```python
from build123d import *

# Parameters (mm, degrees)
ESQUISSE1_W                    = 60
ESQUISSE1_H                    = 35
MAIN_DEPTH                     = 3
ESQUISSE2_W                    = 60
ESQUISSE2_H                    = 2.9
HORIZONTALMAKERBEAMRAIL1_DEPTH = 1
ESQUISSE3_R                    = 1.5
VERTICALFIXHOLE_DEPTH          = 5
ESQUISSE4_W                    = 25
ESQUISSE4_H                    = 25
ESQUISSE4_W_2                  = 18
ESQUISSE4_H_2                  = 18
URGENCYBUTTON_DEPTH            = 20
ESQUISSE5_W                    = 18
ESQUISSE5_H                    = 18
URGENCYBUTTONHOLE_DEPTH        = 1
URGENCYBUTTONHOLE_DEPTH_BACK   = 24
BOSS_EXTRU_4_DEPTH             = 5
ESQUISSE7_W                    = 6
ESQUISSE7_H                    = 25
BOSS_EXTRU_5_DEPTH             = 5
ESQUISSE8_W                    = 29.5
ESQUISSE8_H                    = 10.5
SWITCHHOLE_DEPTH               = 29
ESQUISSE10_W                   = 35
ESQUISSE10_H                   = 16.5
ESQUISSE10_W_2                 = 29.5
ESQUISSE10_H_2                 = 10.5
BOSS_EXTRU_6_DEPTH             = 18
ESQUISSE11_W                   = 35
ESQUISSE11_H                   = 8.5
ENL_V_MAT_EXTRU_4_DEPTH        = 4
ESQUISSE12_W                   = 60
ESQUISSE12_H                   = 2.8
BOSS_EXTRU_7_DEPTH             = 1
BOSS_EXTRU_8_DEPTH             = 60
BOSS_EXTRU_9_DEPTH             = 60


with BuildPart() as part:
    # Esquisse1 → Main (new body)
    with BuildSketch(Plane.XY):
        Rectangle(ESQUISSE1_W, ESQUISSE1_H)
    extrude(amount=MAIN_DEPTH)

    # Esquisse2 → HorizontalMakerBeamRail1 (add)
    with BuildSketch(Plane.XY.offset(3)):
        with Locations((0, 12.5)):
            Rectangle(ESQUISSE2_W, ESQUISSE2_H)
    extrude(amount=HORIZONTALMAKERBEAMRAIL1_DEPTH)

    # Esquisse3 → VerticalFixHole (cut, through all)
    with BuildSketch(Plane(origin=(0, 0, 0), x_dir=(-1, 0, 0), z_dir=(0, 0, -1))):
        with Locations((0, 12.5)):
            Circle(ESQUISSE3_R)
    extrude(amount=-VERTICALFIXHOLE_DEPTH, mode=Mode.SUBTRACT)

    # Esquisse4 → UrgencyButton (add)
    with BuildSketch(Plane.XY.offset(3)):
        with Locations((-17.5, -5)):
            Rectangle(ESQUISSE4_W, ESQUISSE4_H)
        with Locations((-17.5, -5)):
            Rectangle(ESQUISSE4_W_2, ESQUISSE4_H_2, mode=Mode.SUBTRACT)
    extrude(amount=URGENCYBUTTON_DEPTH)

    # Esquisse5 → UrgencyButtonHole (cut, two sides)
    with BuildSketch(Plane.XY.offset(23)) as urgencybuttonhole_sk:
        with Locations((-17.5, -5)):
            Rectangle(ESQUISSE5_W, ESQUISSE5_H)
    extrude(amount=URGENCYBUTTONHOLE_DEPTH, mode=Mode.SUBTRACT)
    extrude(urgencybuttonhole_sk.sketch, amount=-URGENCYBUTTONHOLE_DEPTH_BACK, mode=Mode.SUBTRACT)

    # Esquisse6 → Boss.-Extru.4 (add)
    with BuildSketch(Plane.XY.offset(23)):
        Polygon((-30, -17.5), (-5, -17.5), (-5, 7.5), (-30, 7.5), (-30, 3), (-9.5, 3), (-9.5, -13), (-30, -13), align=None)
    extrude(amount=BOSS_EXTRU_4_DEPTH)

    # Esquisse7 → Boss.-Extru.5 (add)
    with BuildSketch(Plane.XY.offset(28)):
        with Locations((-17.5, -5)):
            Rectangle(ESQUISSE7_W, ESQUISSE7_H)
    extrude(amount=-BOSS_EXTRU_5_DEPTH)

    # Esquisse8 → SwitchHole (cut, through all)
    with BuildSketch(Plane(origin=(0, 0, 0), x_dir=(-1, 0, 0), z_dir=(0, 0, -1))):
        with Locations((-12.25, -0.75)):
            Rectangle(ESQUISSE8_W, ESQUISSE8_H)
    extrude(amount=-SWITCHHOLE_DEPTH, mode=Mode.SUBTRACT)

    # Esquisse10 → Boss.-Extru.6 (add)
    with BuildSketch(Plane.XY.offset(3)):
        with Locations((12.5, -0.75)):
            Rectangle(ESQUISSE10_W, ESQUISSE10_H)
        with Locations((12.25, -0.75)):
            Rectangle(ESQUISSE10_W_2, ESQUISSE10_H_2, mode=Mode.SUBTRACT)
    extrude(amount=BOSS_EXTRU_6_DEPTH)

    # Esquisse11 → Enlèv. mat.-Extru.4 (cut, through all)
    with BuildSketch(Plane.XY.offset(3)):
        with Locations((12.5, -13.25)):
            Rectangle(ESQUISSE11_W, ESQUISSE11_H)
    extrude(amount=-ENL_V_MAT_EXTRU_4_DEPTH, mode=Mode.SUBTRACT)

    # Esquisse12 → Boss.-Extru.7 (add)
    with BuildSketch(Plane(origin=(0, 7.5, 0), x_dir=(1, 0, 0), z_dir=(0, 1, 0))):
        with Locations((0, -8.05)):
            Rectangle(ESQUISSE12_W, ESQUISSE12_H)
    extrude(amount=BOSS_EXTRU_7_DEPTH)

    # Esquisse13 → Boss.-Extru.8 (add, through all)
    with BuildSketch(Plane(origin=(30, 0, 0), x_dir=(0, 0, -1), z_dir=(1, 0, 0))):
        Polygon((-13.1, 7.5), (-13.1, 11.05), (-12.1, 11.05), (-12.1, 13.95), (-13.1, 13.95), (-13.1, 17.5), (-16.1, 17.5), (-16.1, 7.5), align=None)
    extrude(amount=-BOSS_EXTRU_8_DEPTH)

    # Esquisse14 → Boss.-Extru.9 (add, through all)
    with BuildSketch(Plane(origin=(30, 0, 0), x_dir=(0, 0, -1), z_dir=(1, 0, 0))):
        Polygon((-16.1, 7.5), (-16.1, 17.5), (-21, 7.5), align=None)
    extrude(amount=-BOSS_EXTRU_9_DEPTH)


solid = part.part
```
CAD build for the part. Positions are in the model's coordinates, mm. A direction names the side the tool comes from. Round coordinates to 2 decimals unless told otherwise and drop trailing zeros. Write each loop counter-clockwise with the first axis right and the second up, starting at its lowest first coordinate (ties: lowest second). Pieces come first, ordered by that corner, then holes. Notation, with made-up numbers: M 25,89.5 L 75,89.5 A24 cw 75,117.5 Z; hole C 7,83.5 d6. An arc over 180 degrees is marked long. One line per question, with ' | ' between items.
1. Cut at C-C on y = -10.5. Write the cut outline in (x, z), and give its area (4 significant figures).
Working result:
outline: M -30,0 L -26.5,0 L -26.5,23 L -30,23 Z; M -20.5,23 L -14.5,23 L -14.5,28 L -20.5,28 Z; M -9.5,23 L -8.5,23 L -8.5,0 L -5,0 L -5,28 L -9.5,28 Z | area: 213.5 mm2
2. Mould opens along X. For faces 4 (the flat face through (0, 17.5, 15)), 5 (the flat face through (-18, -14, 11)), 6 (the flat face through (30, 1, 11)) say: pulls with the +X half, pulls with the -X half, needs draft (parallel to the pull), parting line crosses it, or undercut.
Working result:
face 4: needs draft | face 5: undercut | face 6: pulls with the +X half
3. Cut at D-D on z = 26.5. Write the cut outline in (x, y), and give its area (3 significant figures).
Working result:
outline: M -30,-17.5 L -5,-17.5 L -5,7.5 L -30,7.5 L -30,3 L -20.5,3 L -20.5,-13 L -30,-13 Z; hole M -14.5,-13 L -9.5,-13 L -9.5,3 L -14.5,3 Z | area: 393 mm2
4. Pin check, flat tips, straight feed: pin 1 Ø1.1 at (x, y) = (14, 8) entering from +Z; pin 2 Ø4 at (y, z) = (12.5, 23) entering from -X; pin 3 Ø1.1 at (x, y) = (-10, 16) entering from +Z; pin 4 Ø3.5 at (x, y) = (0, 12.5) entering from +Z. Stop position of each tip, or through.
Working result:
pin 1: z = 21 | pin 2: through | pin 3: z = 17.1 | pin 4: z = 19.41
5. Which spindle directions (+Z, -Z, +X, -X, +Y, -Y) get a long thin tool onto all of the face, cutting with end or side? Do faces 1 (the flat face through (12, 5, 21)), 2 (the cylindrical face through (-1.386, 11.925, 1.972)), 3 (the flat face through (-2.5, -1, 10)). Say none if no direction does.
Working result:
face 1: +Z, +X, +Y, -Y | face 2: -Z | face 3: +Z, -Z
6. Cut at A-A on x = 14.5. Write the cut outline in (y, z).
Working result:
outline: M -9,0 L -6,0 L -6,21 L -9,21 Z; M 4.5,0 L 17.5,0 L 17.5,3 L 13.95,3 L 13.95,4 L 11.05,4 L 11.05,3 L 7.5,3 L 7.5,6.65 L 8.5,6.65 L 8.5,9.45 L 7.5,9.45 L 7.5,13.1 L 11.05,13.1 L 11.05,12.1 L 13.95,12.1 L 13.95,13.1 L 17.5,13.1 L 17.5,16.1 L 7.5,21 L 4.5,21 Z
7. Probe L1, parallel to Y at x = 0, z = 2.6; L2, parallel to Y at x = 18, z = 3.75; L3, parallel to X at y = -3, z = 5.5. List the from-to ranges inside material, lowest first. Write a range as from..to.
Working result:
L1: -9..-6, 4.5..11, 14..17.5 | L2: -9..-6, 4.5..7.5, 11.05..13.95 | L3: -30..-26.5, -8.5..-2.5, 27..30
8. Cut at B-B on z = 10.5. Write the cut outline in (x, y).
Working result:
outline: M -30,-17.5 L -5,-17.5 L -5,-9 L 30,-9 L 30,7.5 L -30,7.5 Z; hole M -26.5,-14 L -8.5,-14 L -8.5,4 L -26.5,4 Z; hole M -2.5,-6 L 27,-6 L 27,4.5 L -2.5,4.5 Z
